Build history of the part. All positions in model axes, mm. Face numbers are marked on the shaded views. A direction names the side the tool comes from. Round coordinates to 2 decimals unless told otherwise and drop trailing zeros. Loops run counter-clockwise (first coordinate to the right, second up) from the corner with the lowest first, then second, coordinate; pieces in that order, holes last. Notation, with made-up numbers: (-2, 27.25) - (26, 27.25) arc R19 ccw to (26, 48.25) - close; hole circle Ø11 at (5, 12). An arc over 180 degrees is marked (long way). Use one line per item in the form item = value. Start each with the question number.
Q1. Drill centre lines: line 1 (X direction, y = -5, z = 2.1); line 2 (X direction, y = 11, z = 18); line 3 (Z direction, x = 30, y = 15). Where is each one in solid material? Low to high.
Q2. Saw through at B-B (z = 9). Give the cut face in (x, y).
Q3. 3-axis set-ups, long thin cutter, end or side, ignore diameter. For the marked faces 1, 2 and 3: which of +Z, -Z, +X, -X, +Y, -Y reach the whole face in a straight line?
Q4. Pin check, flat tips, straight feed: pin 1 (1 mm diameter, centred on x = -5, y = -8.5, fed in from +Z); pin 2 (1.2 mm diameter, centred on y = -15, z = 20, fed in from +X); pin 3 (1.9 mm diameter, centred on x = 0, y = 9, fed in from +Z); pin 4 (2.5 mm diameter, centred on x = -13.42, y = 5, fed in from +Z). Stop position of each tip, or through.
Q5. Saw through at C-C (x = 16). Give the cut face in (y, z).
Q6. Mould opens along X. For the marked faces 4, 5 and 6 say: released by +X, released by -X, zero draft, split by the parting line, or undercut.
Q7. Saw through at D-D (z = 12.25). Give the cut face in (x, y), then the cut area to 3 significant figures.
Q8. Saw through at A-A (y = -5). Give the cut face in (x, z), then the cut area to 3 significant figures.
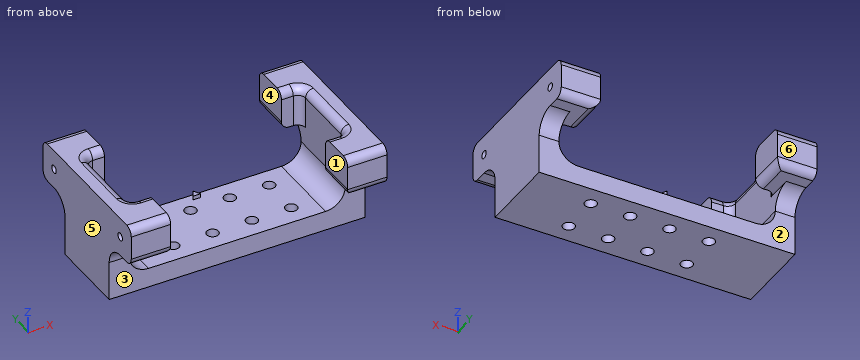
```python
from build123d import *

# Parameters (mm, degrees)
F1_DEPTH    = 10
F4_DEPTH    = 1
F5_W        = 10
F5_H        = 10.0000003353
F6_DEPTH    = 10
F7_D        = 2
F7_DEPTH    = 8
F7_TIP      = 0.600860619
F8_R        = 2
F9_T1_DEPTH = 5
F9_T3_DEPTH = 20
F10_R       = 2
F12_D       = 3
F13_R       = 2


# Not quite as in the source:
# - a fillet or chamfer that OpenCascade refuses, or shapes differently, is made with other operations: its cross-section is extruded or revolved along the edge and cut away or added


with BuildPart() as f1:
    # F0 (on Front) → F1 (new body, symmetric)
    with BuildSketch(Plane.XZ):
        Polygon((-27.5, 25), (-32.5, 25), (-32.5, 0), (32.5, 0), (32.5, 25), (27.5, 25), (27.5, 5), (-27.5, 5), align=None)
    extrude(amount=F1_DEPTH, both=True)

    # F3 (on face) → F4 (join)
    with BuildSketch(Plane.XY.offset(5)):
        Polygon((1, 8.2679491924), (0, 10), (-1, 8.2679491924), align=None)
    extrude(amount=F4_DEPTH)

    # F5 (on face) → F6 (join)
    with BuildSketch(Plane(origin=(-32.5, 0, 0), x_dir=(0, -1, 0), z_dir=(-1, 0, 0))):
        with Locations((-15, 19.9999998324)):
            Rectangle(F5_W, F5_H)
        with Locations((15, 19.9999998324)):
            Rectangle(F5_W, F5_H)
    extrude(amount=-F6_DEPTH)

    # F7
    with Locations(Plane(origin=(-32.5, 0, 0), x_dir=(0, -1, 0), z_dir=(-1, 0, 0))):
        with Locations((-15, 19.9999998324), (15, 19.9999998324)):
            Hole(F7_D / 2, depth=F7_DEPTH)
            with Locations((0, 0, -(F7_DEPTH + F7_TIP / 2))):  # 118° drill point
                Cone(0, F7_D / 2, F7_TIP, mode=Mode.SUBTRACT)

    # F8
    f8_edges = [f1.edges().sort_by_distance(p)[0] for p in [
        (-27.5, -20, 25),
        (-27.5, 20, 25),
        (-27.5, 20, 15),
        (-22.5, 15, 15),
        (-22.5, -15, 15),
        (-27.5, -20, 15),
    ]]
    fillet(f8_edges, radius=F8_R)

    # F9: fillet of radius 5 on 4 edges, made by hand

    # F9_s2 → F9_t1 (join)
    with BuildSketch(Plane.YZ.offset(-32.5)):
        with BuildLine():
            ThreePointArc((-15, 14.9999996647), (-11.4644660941, 13.5355335707), (-10, 9.9999996647))
            Line((-10, 9.9999996647), (-10, 14.9999996647))
            Line((-10, 14.9999996647), (-15, 14.9999996647))
        make_face()
        with BuildLine():
            ThreePointArc((15, 14.9999996647), (11.4644660941, 13.5355335707), (10, 9.9999996647))
            Line((10, 9.9999996647), (10, 14.9999996647))
            Line((10, 14.9999996647), (15, 14.9999996647))
        make_face()
    extrude(amount=F9_T1_DEPTH)

    # F9_s4 → F9_t3 (join)
    with BuildSketch(Plane.XZ.offset(-10)):
        with BuildLine():
            ThreePointArc((-27.5, 10), (-26.0355339059, 6.4644660941), (-22.5, 5))
            Line((-22.5, 5), (-27.5, 5))
            Line((-27.5, 5), (-27.5, 10))
        make_face()
        with BuildLine():
            ThreePointArc((22.5, 5), (26.0355339059, 6.4644660941), (27.5, 10))
            Line((27.5, 10), (27.5, 5))
            Line((27.5, 5), (22.5, 5))
        make_face()
    extrude(amount=F9_T3_DEPTH)

    # F10
    f10_edges = [f1.edges().sort_by_distance(p)[0] for p in [
        (-27.5, 10, 20),
        (-27.5, -10, 20),
    ]]
    fillet(f10_edges, radius=F10_R)

    # F11: F1 across plane


with BuildPart() as f1_1:
    add(f1.part)
    add(f1.part.mirror(Plane.YZ))

    # F12 (through all)
    with Locations(Plane(origin=(0, 0, 0), x_dir=(1, 0, 0), z_dir=(0, 0, -1))):
        with Locations((-13.4210362619, 5.0000001118), (-3.4210362619, 5.0000001118), (6.5789637381, 5.0000001118), (16.5789637381, 5.0000001118), (-13.4210362619, -4.9999998882), (-3.4210362619, -4.9999998882), (6.5789637381, -4.9999998882), (16.5789637381, -4.9999998882)):
            Hole(F12_D / 2)

    # F13
    f13_edges = [f1_1.edges().sort_by_distance(p)[0] for p in [
        (-27.5, 0, 25),
        (27.5, 0, 25),
        (-24, -10, 25),
        (-26.914214, -9.414214, 25),
        (-26.914214, 9.414214, 25),
        (-24, 10, 25),
        (24, 10, 25),
        (26.914214, 9.414214, 25),
        (26.914214, -9.414214, 25),
        (24, -10, 25),
    ]]
    fillet(f13_edges, radius=F13_R)


solid = f1_1.part
```
Report:
q1.line_1 = -32.5 to -14.92, -11.92 to -4.92, -1.92 to 5.08, 8.08 to 15.08, 18.08 to 32.5
q1.line_2 = -32.5 to -22.5, 22.5 to 32.5
q1.line_3 = 15 to 19, 21 to 25
q2.outline = (-32.5, -10) - (-27.4, -10) - (-27.4, 10) - (-32.5, 10) - close; (27.4, -10) - (32.5, -10) - (32.5, 10) - (27.4, 10) - close
q3.face_1 = +Z, -Z, +Y, -Y
q3.face_2 = -Z, +X, -X, +Y
q3.face_3 = -Z, +X, -X, -Y
q4.pin_1 = 5
q4.pin_2 = 24.26
q4.pin_3 = 6
q4.pin_4 = through
q5.outline = (-10, 0) - (-6.38, 0) - (-6.38, 5) - (-10, 5) - close; (-3.62, 0) - (3.62, 0) - (3.62, 5) - (-3.62, 5) - close; (6.38, 0) - (10, 0) - (10, 5) - (6.38, 5) - close
q6.face_4 = undercut
q6.face_5 = released by -X
q6.face_6 = zero draft
q7.outline = (-32.5, -10.53) - (-27.5, -10.53) - (-27.5, 10.53) - (-32.5, 10.53) - close; (27.5, -10.53) - (32.5, -10.53) - (32.5, 10.53) - (27.5, 10.53) - close
q7.area = 211 mm²
q8.outline = (-32.5, 0) - (-14.92, 0) - (-14.92, 5) - (-22.5, 5) arc R5 cw to (-27.5, 10) - (-27.5, 23) arc R2 ccw to (-29.5, 25) - (-32.5, 25) - close; (-11.92, 0) - (-4.92, 0) - (-4.92, 5) - (-11.92, 5) - close; (-1.92, 0) - (5.08, 0) - (5.08, 5) - (-1.92, 5) - close; (8.08, 0) - (15.08, 0) - (15.08, 5) - (8.08, 5) - close; (18.08, 0) - (32.5, 0) - (32.5, 25) - (29.5, 25) arc R2 ccw to (27.5, 23) - (27.5, 10) arc R5 cw to (22.5, 5) - (18.08, 5) - close
q8.area = 474 mm²
